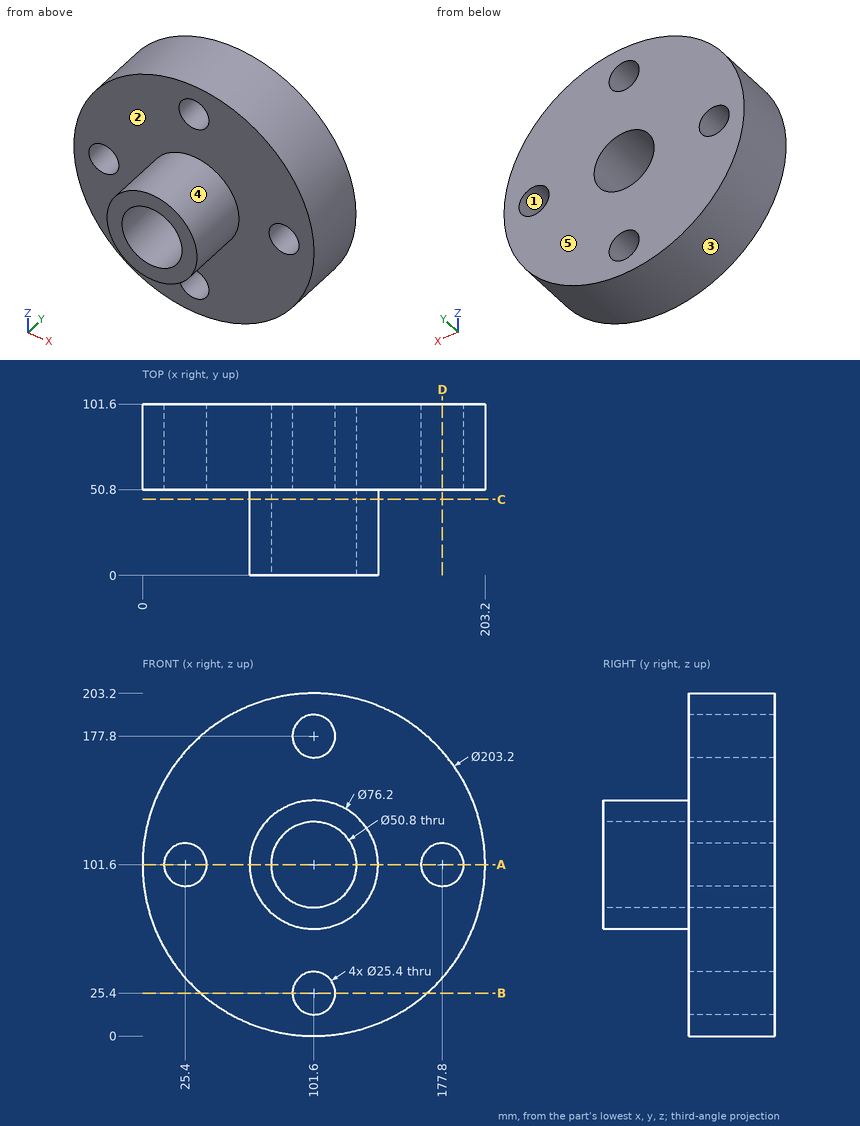
Here's the drawing with two shaded views (mm, measured from the low corner). I have some questions. A direction names the side the tool comes from. Round coordinates to 2 decimals unless told otherwise and drop trailing zeros. Write each loop counter-clockwise with the first axis right and the second up, starting at its lowest first coordinate (ties: lowest second). Pieces come first, ordered by that corner, then holes. Notation, with made-up numbers: M 74,30 L 110,30 A4 ccw 110,34 Z; hole C 74.25,80 d5. An arc over 180 degrees is marked long. Use CSV: the item, a comma, the result in double quotes.
(1) On a 3-axis mill with a long thin cutter (end or side, diameter ignored), from which of +Z, -Z, +X, -X, +Y, -Y can I reach the whole of each face in a straight line? I mean the marked faces 4 and 5. Say none if no direction works.
Check values:
face 4,"-Y"
face 5,"+Z, -Z, +X, -X, +Y"
(2) I need wall thicknesses on line 1 along Z through (x, y) = (101, 88); line 2 along Z through (x, y) = (101.6, 50.5); line 3 along X through (y, z) = (63.5, 106.5). Which ranges of each line are inside material? Lowest first, please.
Check values:
line 1,"0 to 12.71, 38.09 to 76.21, 126.99 to 165.11, 190.49 to 203.2"
line 2,"63.5 to 76.2, 127 to 139.7"
line 3,"0.12 to 13.68, 37.12 to 76.68, 126.52 to 166.08, 189.52 to 203.08"
(3) I'm going to push flat-ended pins straight in: pin 1 (12 mm diameter, centred on y = 71.5, z = 73.5, fed in from -X); pin 2 (23 mm diameter, centred on x = 101.6, z = 25.4, fed in from -Y); pin 3 (4 mm diameter, centred on x = 38.5, y = 85, fed in from +Z); pin 4 (4 mm diameter, centred on y = 58.5, z = 180.5, fed in from +X). Where does each tip first touch, or does it pass through?
Check values:
pin 1,"x = 2.43"
pin 2,"through"
pin 3,"z = 182.77"
pin 4,"x = 168"
(4) Imagine slicing it at B-B (z = 25.4). Write out the boundary of the cut face in (x, y), plus the area to 3 significant figures.
Check values:
outline,"M 34.4,50.8 L 88.9,50.8 L 88.9,101.6 L 34.4,101.6 Z; M 114.3,50.8 L 168.8,50.8 L 168.8,101.6 L 114.3,101.6 Z"
area,"5,540 mm^2"
(5) Imagine slicing it at C-C (y = 45). Write out the boundary of the cut face in (x, z).
Check values:
outline,"C 101.6,101.6 d76.2; hole C 101.6,101.6 d50.8"
(6) Imagine slicing it at D-D (x = 177.8). Write out the boundary of the cut face in (y, z), plus the area to 3 significant figures.
Check values:
outline,"M 50.8,34.4 L 101.6,34.4 L 101.6,88.9 L 50.8,88.9 Z; M 50.8,114.3 L 101.6,114.3 L 101.6,168.8 L 50.8,168.8 Z"
area,"5,540 mm^2"
(7) Imagine slicing it at A-A (z = 101.6). Write out the boundary of the cut face in (x, y).
Check values:
outline,"M 0,50.8 L 12.7,50.8 L 12.7,101.6 L 0,101.6 Z; M 38.1,50.8 L 63.5,50.8 L 63.5,0 L 76.2,0 L 76.2,101.6 L 38.1,101.6 Z; M 127,0 L 139.7,0 L 139.7,50.8 L 165.1,50.8 L 165.1,101.6 L 127,101.6 Z; M 190.5,50.8 L 203.2,50.8 L 203.2,101.6 L 190.5,101.6 Z"
(8) We'd pull the mould along Z, two halves only. Please class the marked faces 1, 2 and 3: +Z half, -Z half, draft (parallel to the pull), parting line (faces both ways), or undercut.
Check values:
face 1,"undercut"
face 2,"draft"
face 3,"parting line"
